Can you work these out from the model? Positions are in its coordinate system, mm. A direction names the side the tool comes from. Coordinates: 2 decimals unless noted, no trailing zeros. Order: outer loops, then holes, each group sorted by start corner. A loop starts at its lowest first (then second) coordinate and runs counter-clockwise, first axis right, second up. Notation, with made-up numbers: (-39.75, -23.75) -> (-16.75, -23.75) arc R20 ccw to (-16.75, -6.75) -> close; hole circle Ø10 at (19.5, 4.5). An arc over 180 degrees is marked (long way). Write item = value, one per line. Start each with the question number.
from build123d import *

# Parameters (mm, degrees)
SKETCH1_R                    = 38.5
SKETCH1_R_2                  = 1
BASE_FLANGE1_DEPTH           = 3
EDGE_FLANGE1_STRIP_W         = 18
EDGE_FLANGE1_STRIP_H         = 3
EDGE_FLANGE1_STRIP_CUT_DEPTH = 92
EDGE_FLANGE1_DEPTH           = 92
EDGE_FLANGE1_START           = 3
EDGE_FLANGE1_PROFILE_W       = 92
EDGE_FLANGE1_PROFILE_H       = 17.5
EDGE_FLANGE1_PROFILE_R       = 1
EDGE_FLANGE1_FLAT_DEPTH      = 3
FILLET1_R                    = 2
M3_CLEARANCE_HOLE1_D         = 3.2
M3_CLEARANCE_HOLE1_DEPTH     = 136
M3_CLEARANCE_HOLE1_TIP       = 0.96137699
M5_CLEARANCE_HOLE1_D         = 5.3
M5_CLEARANCE_HOLE1_DEPTH     = 136
M5_CLEARANCE_HOLE1_TIP       = 1.59228064


# Sheet-metal steps are written as plain solids
with BuildPart() as part:
    # Sketch1 → Base-Flange1 (new body)
    with BuildSketch(Plane(origin=(0, 0, 0), x_dir=(1, 0, 0), z_dir=(0, 1, 0))):
        with BuildLine():
            Line((-46, 0), (-46, -55))
            Line((-46, -55), (46, -55))
            Line((46, -55), (46, 0))
            ThreePointArc((46, 0), (0, 46), (-46, 0))
        make_face()
        with Locations(Location((0, 0, 0), (0, 0, 270))):
            Circle(SKETCH1_R, mode=Mode.SUBTRACT)
        with Locations(Location((0, 41.5, 0), (0, 0, 270))):
            Circle(SKETCH1_R_2, mode=Mode.SUBTRACT)
        with Locations(Location((29.344931419, 29.344931419, 0), (0, 0, 270))):
            Circle(SKETCH1_R_2, mode=Mode.SUBTRACT)
        with Locations(Location((41.5, 0, 0), (0, 0, 270))):
            Circle(SKETCH1_R_2, mode=Mode.SUBTRACT)
        with Locations(Location((29.344931419, -29.344931419, 0), (0, 0, 270))):
            Circle(SKETCH1_R_2, mode=Mode.SUBTRACT)
        with Locations(Location((0, -41.5, 0), (0, 0, 270))):
            Circle(SKETCH1_R_2, mode=Mode.SUBTRACT)
        with Locations(Location((-29.344931419, -29.344931419, 0), (0, 0, 270))):
            Circle(SKETCH1_R_2, mode=Mode.SUBTRACT)
        with Locations(Location((-41.5, 0, 0), (0, 0, 270))):
            Circle(SKETCH1_R_2, mode=Mode.SUBTRACT)
        with Locations(Location((-29.344931419, 29.344931419, 0), (0, 0, 270))):
            Circle(SKETCH1_R_2, mode=Mode.SUBTRACT)
    extrude(amount=-BASE_FLANGE1_DEPTH)

    # Edge-Flange1 strip (across the edge) → Edge-Flange1 strip cut (cut)
    with BuildSketch(Plane(origin=(-46, 0, 55), x_dir=(0, 0, -1), z_dir=(1, 0, 0))):
        with Locations((-6, -1.5)):
            Rectangle(EDGE_FLANGE1_STRIP_W, EDGE_FLANGE1_STRIP_H)
    extrude(amount=EDGE_FLANGE1_STRIP_CUT_DEPTH, mode=Mode.SUBTRACT)

    # Edge-Flange1 bend section (across the edge) → Edge-Flange1 (add)
    with BuildSketch(Plane(origin=(-46, 0, 55), x_dir=(0, 0, -1), z_dir=(1, 0, 0))):
        with BuildLine():
            Line((-3, 3), (0, 3))
            ThreePointArc((0, 3), (0.878679656, 0.878679656), (3, 0))
            Line((3, 0), (3, -3))
            ThreePointArc((3, -3), (-1.242640687, -1.242640687), (-3, 3))
        make_face()
    extrude(amount=EDGE_FLANGE1_DEPTH)

    # Edge-Flange1 profile (on flange) → Edge-Flange1 flat (add)
    with BuildSketch(Plane.XY.offset(55).offset(EDGE_FLANGE1_START)):
        with Locations((0, 11.75)):
            Rectangle(EDGE_FLANGE1_PROFILE_W, EDGE_FLANGE1_PROFILE_H)
        with Locations((-30, 9.8)):
            Circle(EDGE_FLANGE1_PROFILE_R, mode=Mode.SUBTRACT)
        with Locations((30, 9.8)):
            Circle(EDGE_FLANGE1_PROFILE_R, mode=Mode.SUBTRACT)
    extrude(amount=-EDGE_FLANGE1_FLAT_DEPTH)

    # Fillet1
    fillet1_edges = [part.edges().sort_by_distance(p)[0] for p in [
        (-46, 20.5, 56.5),
        (46, 20.5, 56.5),
    ]]
    fillet(fillet1_edges, radius=FILLET1_R)

    # M3 Clearance Hole1
    with Locations(Plane(origin=(0, 0, 0), x_dir=(1, 0, 0), z_dir=(0, 1, 0))):
        with Locations((-29.344931419, 29.344931419), (0, 41.5), (-41.5, 0), (-29.344931419, -29.344931419), (0, -41.5), (29.344931419, -29.344931419), (41.5, 0), (29.344931419, 29.344931419)):
            Hole(M3_CLEARANCE_HOLE1_D / 2, depth=M3_CLEARANCE_HOLE1_DEPTH)
            with Locations((0, 0, -(M3_CLEARANCE_HOLE1_DEPTH + M3_CLEARANCE_HOLE1_TIP / 2))):  # 118° drill point
                Cone(0, M3_CLEARANCE_HOLE1_D / 2, M3_CLEARANCE_HOLE1_TIP, mode=Mode.SUBTRACT)

    # M5 Clearance Hole1
    with Locations(Plane.XY.offset(58)):
        with Locations((-30, 9.8), (30, 9.8)):
            Hole(M5_CLEARANCE_HOLE1_D / 2, depth=M5_CLEARANCE_HOLE1_DEPTH)
            with Locations((0, 0, -(M5_CLEARANCE_HOLE1_DEPTH + M5_CLEARANCE_HOLE1_TIP / 2))):  # 118° drill point
                Cone(0, M5_CLEARANCE_HOLE1_D / 2, M5_CLEARANCE_HOLE1_TIP, mode=Mode.SUBTRACT)


solid = part.part
(1) Thinking about a two-plate mould opening in X: for faces 3 (the face through (-21, -3, 35)), 4 (the face through (1.01, -1.48, -45.99)), 5 (the face through (-0.74, -1.52, 42.92)), which applies, +X half, -X half, draft (parallel to the pull), parting line (faces both ways), or undercut?
(2) For faces 1 (the face through (46, -0.3, 33.4)), 2 (the face through (-21, 0, 35)), which set-ups out of +Z, -Z, +X, -X, +Y, -Y let a thin tool reach every point of the face, with its end or its side?
(3) Imagine slicing it at B-B (x = -7.5). Write out the boundary of the cut face in (y, z).
(4) Imagine slicing it at D-D (x = 35). Write out the boundary of the cut face in (y, z), plus the area to 3 significant figures.
(5) For P1, Ø5, axis at y = 2, z = -9, coming from the +X side; P2, Ø3.5, axis at x = -29.34, z = -29.34, coming from the +Y side; P3, Ø6, axis at x = -10, y = 12.5, coming from the -Z side; P4, Ø4, axis at x = -41.5, z = 0, coming from the -Y side, each with a flat end and sliding along its axis, tell me the tip position at first contact or that it passes through.
(6) Imagine slicing it at A-A (z = -41.5). Write out the boundary of the cut face in (x, y), plus the area to 3 significant figures.
(7) If I drill on L1, parallel to X at y = -0.5, z = 28; L2, parallel to Y at x = 26, z = -32.5; L3, parallel to Z at x = 15, y = 15.25, over which ranges is the centre line in solid material (lowest first)? Write a range as from..to.
(8) Imagine slicing it at C-C (z = 9). Write out the boundary of the cut face in (x, y), plus the area to 3 significant figures.
Result set:
q1.face_3 = draft
q1.face_4 = parting line
q1.face_5 = undercut
q2.face_1 = +Z, -Z, +X, +Y, -Y
q2.face_2 = -Z, +X, -X, +Y
q3.outline = (-3, -45.38) -> (0, -45.38) -> (0, -37.76) -> (-3, -37.76) -> close; (-3, 37.76) -> (0, 37.76) -> (0, 52) arc R3 cw to (3, 55) -> (20.5, 55) -> (20.5, 58) -> (3, 58) arc R6 ccw to (-3, 52) -> close
q4.outline = (-3, -29.85) -> (0, -29.85) -> (0, -16.04) -> (-3, -16.04) -> close; (-3, 16.04) -> (0, 16.04) -> (0, 52) arc R3 cw to (3, 55) -> (20.5, 55) -> (20.5, 58) -> (3, 58) arc R6 ccw to (-3, 52) -> close
q4.area = 223 mm2
q5.P1 = 45.38
q5.P2 = 0
q5.P3 = 55
q5.P4 = -3
q6.outline = (-19.84, -3) -> (-1.6, -3) -> (-1.6, 0) -> (-19.84, 0) -> close; (1.6, -3) -> (19.84, -3) -> (19.84, 0) -> (1.6, 0) -> close
q6.area = 109 mm2
q7.L1 = -46..-30.21, -28.48..-26.42, 26.42..28.48, 30.21..46
q7.L2 = -3..0
q7.L3 = 55..58
q8.outline = (-46, -3) -> (-37.43, -3) -> (-37.43, 0) -> (-46, 0) -> close; (37.43, -3) -> (46, -3) -> (46, 0) -> (37.43, 0) -> close
q8.area = 51.4 mm2
